The listing builds one solid part. Answer for the finished solid, in the listing's coordinates (mm). A direction names the side the tool comes from. Round coordinates to 2 decimals unless told otherwise and drop trailing zeros. Write each loop counter-clockwise with the first axis right and the second up, starting at its lowest first coordinate (ties: lowest second). Pieces come first, ordered by that corner, then holes.
(1) For faces 1 (the face through (-920.75, -7, 25)), 2 (the face through (-923.925, -7, 26)), determine the directions among +Z, -Z, +X, -X, +Y, -Y from which every point of the face is accessible in a straight line to the end or side of a thin tool.
(2) A cutting plane is placed at B-B, the plane z = 31.5. Give the vertices of the cut face in (x, y) (3 decimals).
(3) Find the intervals of material crossed by probe 1 along X at (y, z) = (126, 20); probe 2 along Z at (x, y) = (-918.5, -147) (3 decimals); probe 3 along Z at (x, y) = (-921, -231), in increasing order.
(4) A cutting plane is placed at C-C, the plane x = -897. Give the vertices of the cut face in (y, z) (3 decimals).
(5) Each of these flat-tipped pins is pushed along its axis until it touches: pin 1 Ø12 at (y, z) = (-195.5, 44.5) entering from +X; pin 2 Ø5 at (x, y) = (-895.5, -160.5) entering from +Z (3 decimals). Where does it stop, or does it pass through?
(6) A cutting plane is placed at A-A, the plane y = -149.5. Give the vertices of the cut face in (x, z) (3 decimals), and give its area (3 significant figures).
from build123d import *

# Parameters (mm, degrees)
F1_DEPTH = 508
F3_DEPTH = 50.8


# Not quite as in the source:
# - a pattern or mirror of a feature is missing from the dataset's text; its kind, count and spacing are read off the source's solid


with BuildPart() as f1:
    # F0 (on Front) → F1 (new body, symmetric)
    with BuildSketch(Plane.XZ):
        with BuildLine():
            ThreePointArc((-920.7500404358, 47.625), (-921.6799764055, 49.8700640303), (-923.9250404358, 50.8))
            Line((-923.9250404358, 50.8), (-923.9250404358, 0))
            Line((-923.9250404358, 0), (-873.1250404358, 0))
            ThreePointArc((-873.1250404358, 0), (-874.0549764055, 2.2450640303), (-876.3000404358, 3.175))
            Line((-876.3000404358, 3.175), (-920.7500404358, 3.175))
            Line((-920.7500404358, 3.175), (-920.7500404358, 47.625))
        make_face()
    extrude(amount=F1_DEPTH, both=True)

    # F2 (on face) → F3 (cut)
    with BuildSketch(Plane(origin=(0, 0, 0), x_dir=(1, 0, 0), z_dir=(0, 0, -1))):
        Polygon((-873.1250404358, -457.2), (-923.9250404358, -508), (-873.1250404358, -508), align=None)
    f3 = extrude(amount=-F3_DEPTH, mode=Mode.SUBTRACT)

    # F3_copies: F3 across plane
    add(f3.mirror(Plane(origin=(0, 0, 0), x_dir=(0, 0, -1), z_dir=(0, -1, 0))), mode=Mode.SUBTRACT)


solid = f1.part
Solutions:
1. face 1: +Z, +X, +Y, -Y
1. face 2: +Z, -Z, -X, +Y, -Y
2. outline: (-923.925, -508) - (-920.75, -504.825) - (-920.75, 504.825) - (-923.925, 508) - close
3. probe 1: x = -923.93 to -920.75
3. probe 2: z = 0 to 3.175
3. probe 3: z = 0 to 48.86
4. outline: (-481.075, 0) - (481.075, 0) - (481.075, 3.175) - (-481.075, 3.175) - close
5. pin 1: stops at x = -920.75
5. pin 2: stops at z = 3.175
6. outline: (-923.925, 0) - (-873.125, 0) arc R3.175 ccw to (-876.3, 3.175) - (-920.75, 3.175) - (-920.75, 47.625) arc R3.175 ccw to (-923.925, 50.8) - close
6. area: 308 mm2
